Autodesk Inventor part; units mm, degrees
ref_plane "YZ Plane" through (0, 0, 0) normal (1, 0, 0) x (0, 1, 0)
ref_plane "XZ Plane" through (0, 0, 0) normal (0, 1, 0) x (-1, 0, 0)
ref_plane "XY Plane" through (0, 0, 0) normal (0, 0, 1) x (1, 0, 0)
sketch "Sketch1" plane through (0, 0, 0) normal (0, 1, 0) x (-1, 0, 0)
  line L0 (-22.5529, -44.0141) -> (22.4471, -44.0141)
  line L1 (-22.5529, -44.0141) -> (22.4471, -44.0141)
  line L2 (22.4471, 2.9859) -> (22.4471, -44.0141)
  line L3 (22.4471, 2.9859) -> (12.4471, 2.9859)
  line L4 (-22.5529, 2.9859) -> (-22.5529, -44.0141)
  line L5 (-22.5529, 2.9859) -> (-12.4471, 2.9859)
  arc A0 (-12.4471, 2.9859) -> (12.4471, 2.9859) centre (0, 4.1349) ccw
  circle A1 centre (-18.0529, -7.0141) radius 1.95
  circle A2 centre (-18.0529, -7.0141) radius 1.95
  circle A3 centre (17.9471, -7.0141) radius 1.95
  circle A4 centre (17.9471, -7.0141) radius 1.95
  circle A5 centre (0, -32.0141) radius 5.1
  circle A6 centre (-18.0529, -24.0142) radius 2
  circle A7 centre (-18, -40.0141) radius 2
  circle A8 centre (18, -40.0141) radius 2
  circle A9 centre (17.9471, -24.0142) radius 2
  line L6 (0, 4.1349) -> (0, -32.0141) construction
  point P0 (0, 0)
  dimension "d0" = 45
  dimension "d3" = 10
  dimension "d4" = 12.5
  dimension "d7" = 4.5
  dimension "d8" = 10
  dimension "d9" = 12
  dimension "d10" = 4
  dimension "d11" = 16
  dimension "d12" = 36
  dimension "d13" = 16
  dimension "d14" = 4.5
  dimension "d15" = 18
  dimension "d17" = 4.5
  dimension "d19" = 4
  dimension "d20" = 4
  dimension "d21" = 4
  dimension "d22" = 4
  dimension "d23" = 4
  dimension "d29" = 47
  dimension "d33" = 4.5
  dimension "d34" = 10
extrude "Extrusion1" add sketch "Sketch1" along normal blind 5
fillet "Fillet3" [suppressed]
fillet "Fillet4" [suppressed]
sketch "Sketch5" plane through (0, 5, 0) normal (0, 1, 0) x (1, 0, 0)
  arc A0 (12.4471, -2.9859) -> (-12.4471, -2.9859) centre (0, -4.1349) ccw
  arc A1 (12.4471, -2.9859) -> (-12.4471, -2.9859) centre (0, -4.1349) ccw
  line L0 (12.4471, -2.9859) -> (-12.4471, -2.9859)
  circle A2 centre (18.0529, 7.0141) radius 1.95
  circle A3 centre (18.0529, 7.0141) radius 1.95
  circle A4 centre (-17.9471, 7.0141) radius 1.95
  circle A5 centre (-17.9471, 7.0141) radius 1.95
  point P0 (0, 0)
extrude "Extrusion4" add sketch "Sketch5" against normal blind 5
sketch "Sketch8" plane through (0, 5, 0) normal (0, 1, 0) x (1, 0, 0)
  arc A0 (-25.3055, 28.046) -> (25.3055, 28.046) centre (0, 32) ccw
  arc A1 (-34.2883, 25.0481) -> (34.2883, 25.0481) centre (0, 32) ccw
  line L0 (-22.4471, -2.9859) -> (22.5529, -2.9859)
  line L1 (-22.4471, 44.0141) -> (-22.4471, -2.9859)
  line L2 (-22.4471, 29) -> (-34.2883, 25.0481)
  circle A2 centre (0, 32.0141) radius 5.1
  line L3 (0, 32.0141) -> (0, 0) construction
  line L4 (-22.4471, 29) -> (-22.4471, 19.666)
  line L5 (34.2883, 25.0481) -> (22.5529, 29)
  line L6 (22.5529, -2.9859) -> (22.5529, 44.0141)
  line L7 (22.5529, 29) -> (22.5529, 19.8606)
extrude "Extrusion5" add sketch "Sketch8" against normal blind 5 contours L2 L1 A0 | A0 L1 A1 L2 | A0 L6 A1 L1 | L6 L5 A1
sketch "Sketch9" plane through (0, 5, 0) normal (0, 1, 0) x (1, 0, 0)
  circle A0 centre (0, 32) radius 34.9859
  line L0 (-22.4471, -2.9859) -> (22.5529, -2.9859)
  line L1 (22.5529, -2.9859) -> (22.5529, 5.2534)
  line L2 (22.5529, 5.2534) -> (22.5529, -2.9859)
  line L3 (22.5529, -2.9859) -> (-22.4471, -2.9859)
  line L4 (-22.4471, -2.9859) -> (-22.4471, 5.1645)
  point P0 (0, 0)
  point P1 (0, -2.9859)
sketch "Sketch6" plane through (0, 5, 0) normal (0, 1, 0) x (1, 0, 0)
  circle A0 centre (0, 32.0141) radius 5.1
  circle A1 centre (0, 32.0141) radius 32.5 construction
  line L0 (0, 32.0141) -> (0, -0.4859) construction
  line L1 (0, 32.0141) -> (-13.7351, 2.5591) construction
  line L2 (0, 32.0141) -> (-29.455, 18.279) construction
  circle A2 centre (-13, 2.2273) radius 6
  circle A3 centre (-29.455, 18.279) radius 6
  circle A4 centre (13, 2.2273) radius 6
  circle A5 centre (29.455, 18.279) radius 6
  point P0 (0, 0)
  dimension "d49" = 65
  dimension "d50" = 12
  dimension "d51" = 12
  dimension "d52" = 25
  dimension "d53" = 40
extrude "Extrusion6" cut sketch "Sketch9" against normal blind 5 contours A0 L0 L4 | L1 L0 A0
extrude "Extrusion7" cut sketch "Sketch6" against normal blind 5 contours A2 | A3 | A4 | A5
sketch "Sketch10" plane through (0, 5, 0) normal (0, 1, 0) x (1, 0, 0)
  arc A0 (18.9875, 2.6148) -> (8.6459, -1.9008) centre (13, 2.2273) ccw
  circle A1 centre (13, 2.2273) radius 8.25 construction
  arc A2 (-8.6459, -1.9008) -> (-18.9875, 2.6148) centre (-13, 2.2273) ccw
  circle A3 centre (-13, 2.2273) radius 8.25 construction
  arc A4 (-28.9147, 12.3034) -> (-33.6819, 22.5373) centre (-29.455, 18.279) ccw
  circle A5 centre (-29.455, 18.279) radius 8.25 construction
  arc A6 (33.6819, 22.5373) -> (28.9147, 12.3034) centre (29.455, 18.279) ccw
  circle A7 centre (29.455, 18.279) radius 8.25 construction
  circle A8 centre (0, 32.0141) radius 5.1
  circle A9 centre (0, 32.0141) radius 30 construction
  circle A10 centre (21.2132, 10.8009) radius 1.5
  circle A11 centre (0, 2.0141) radius 1.5
  circle A12 centre (-21.2132, 10.8009) radius 1.5
  line L0 (21.2132, 10.8009) -> (0, 32.0141) construction
  line L1 (0, 32.0141) -> (0, 2.0141) construction
  line L2 (0, 32.0141) -> (-21.2132, 10.8009) construction
  point P0 (0, 0)
  dimension "d60" = 16.5
  dimension "d61" = 16.5
  dimension "d62" = 16.5
  dimension "d63" = 16.5
  dimension "d64" = 60
  dimension "d65" = 3
  dimension "d66" = 3
  dimension "d67" = 3
  dimension "d68" = 45
extrude "Extrusion8" cut sketch "Sketch10" against normal blind 10 contours A10 | A11 | A12
sketch "Sketch11" plane through (0, 5, 0) normal (0, 1, 0) x (1, 0, 0)
  line L0 (22.5529, 29) -> (22.5529, 44.0141)
  arc A0 (-22.4471, 29) -> (22.5529, 29) centre (0.0529, 33.7697) ccw
  line L1 (22.5529, 29) -> (22.5529, 44.0141)
  line L2 (22.5529, 44.0141) -> (-22.4471, 44.0141)
  line L3 (-22.4471, 44.0141) -> (-22.4471, 29)
  point P0 (0, 0)
  dimension "d71" = 23
extrude "Extrusion9" cut sketch "Sketch11" against normal blind 10
properties part number "Plunger Holder"
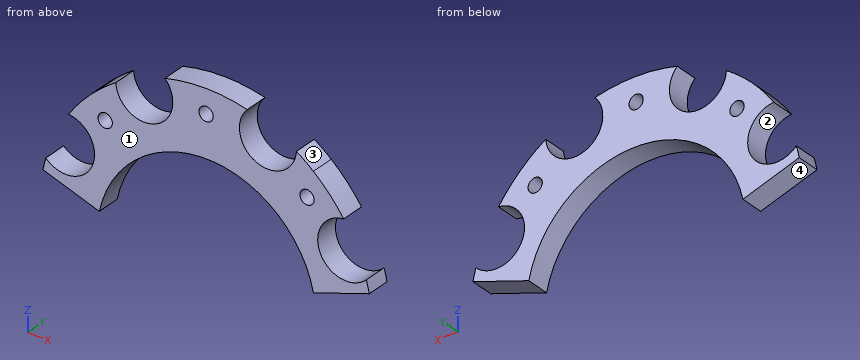
The model under review builds one solid part; all positions refer to its coordinate system, in mm. Face numbers are marked on the shaded views. Give positions to 0.01 mm unless a question says otherwise; leave off trailing zeros. Write each loop counter-clockwise with the first axis right and the second up, starting at its lowest first coordinate (ties: lowest second). Pieces come first, ordered by that corner, then holes. Notation, with made-up numbers: (30, 21.25) -> (36, 21.25) arc R26 cw to (36, 47.25) -> close; hole circle Ø9 at (35, -35.75). An arc over 180 degrees is marked (long way). Answer in a Markdown table with one row per item.
1) Add section C-C on x = 0. State the section outline as (y, z) points.
Worked answers:
| item | result |
|---|---|
| outline | (0, -10.77) -> (5, -10.77) -> (5, -3.51) -> (0, -3.51) -> close; (0, -0.51) -> (5, -0.51) -> (5, 2.99) -> (0, 2.99) -> close |
2) Add section B-B on y = 2.4. State the section outline as (x, z) points (1 decimal), plus the area to 3 significant figures.
Worked answers:
| item | result |
|---|---|
| outline | (-34.3, -25) -> (-22.4, -29) arc R23 cw to (22.6, -29) -> (34.3, -25) arc R35 ccw to (33.7, -22.5) arc R6 cw (long way) to (28.9, -12.3) arc R35 ccw to (19, -2.6) arc R6 cw (long way) to (8.6, 1.9) arc R35 ccw to (-8.6, 1.9) arc R6 cw (long way) to (-19, -2.6) arc R35 ccw to (-22.4, -5.2) arc R35 ccw to (-28.9, -12.3) arc R6 cw (long way) to (-33.7, -22.5) arc R35 ccw to start; hole circle Ø3 at (-21.2, -10.8); hole circle Ø3 at (0, -2); hole circle Ø3 at (21.2, -10.8) |
| area | 694 mm² |
3) Add section D-D on z = -4.5. State the section outline as (x, y) points, plus the area to 3 significant figures.
Worked answers:
| item | result |
|---|---|
| outline | (-21.63, 0) -> (-18.55, 0) -> (-18.55, 5) -> (-21.63, 5) -> close; (-7.45, 0) -> (7.45, 0) -> (7.45, 5) -> (-7.45, 5) -> close; (18.55, 0) -> (21.63, 0) -> (21.63, 5) -> (18.55, 5) -> close |
| area | 105 mm² |
4) For L1, parallel to Z at x = 0, y = 3; L2, parallel to X at y = 2.8, z = -5; L3, parallel to X at y = 3.2, z = -25, list the stretches that pass through material, from the lowest coordinate up. Write a range as [from, to].
Worked answers:
| item | result |
|---|---|
| L1 | [-10.77, -3.51], [-0.51, 2.99] |
| L2 | [-22.25, -18.32], [-7.68, 7.68], [18.32, 22.25] |
| L3 | [-34.28, -21.21], [21.32, 34.28] |
5) Add section A-A on z = -13.5. State the section outline as (x, y) points.
Worked answers:
| item | result |
|---|---|
| outline | (-25.83, 0) -> (-10.82, 0) -> (-10.82, 5) -> (-25.83, 5) -> close; (10.92, 0) -> (25.83, 0) -> (25.83, 5) -> (10.92, 5) -> close |
6) Mouldability with a two-part tool opening along X and no side actions: class the marked faces 1, 2, 3 and 4 as +X half, -X half, draft (parallel to the pull), parting line (faces both ways), or undercut.
Worked answers:
| item | result |
|---|---|
| face 1 | draft |
| face 2 | undercut |
| face 3 | +X half |
| face 4 | -X half |
7) Clearance check with flat-ended pins moving along their axes: P1, Ø1.5, axis at y = 2.5, z = -10, coming from the +X side; P2, Ø11, axis at x = 13, z = -2.23, coming from the -Y side. State where each tip first meets the part, or that it passes through.
Worked answers:
| item | result |
|---|---|
| P1 | x = 27.79 |
| P2 | through |
